```python
from build123d import *

# Parameters (mm, degrees)
POCKET001_DEPTH         = 8
FILLET_R                = 1.5
SKETCH021_R             = 2
POCKET006_DEPTH         = 8
BODY003_PLACEMENT_ANGLE = 127.1


with BuildPart() as part:
    # Sketch009 → Revolution002 (revolve)
    with BuildSketch(Plane.XZ):
        Polygon((35.8, -1.2), (0, -1.2), (0, 0), (37, 0), (37, -2.8), (37, -3.8), (42.222646, -15), (26, -15), (26, -13), (35.8, -3.2), align=None)
    revolve(axis=Axis((0, 0, 0), (0, 0, 1)))

    # Sketch010 (on Face6 of Revolution002) → Pocket001 (cut)
    with BuildSketch(Plane(origin=(0, 0, -15), x_dir=(1, 0, 0), z_dir=(0, 0, -1))):
        with BuildLine():
            ThreePointArc((-4.991228, 41.926596), (0, 37.222646), (4.991228, 41.926596))
            ThreePointArc((4.991228, 41.926596), (0, 42.222646), (-4.991228, 41.926596))
        make_face()
    extrude(amount=-POCKET001_DEPTH, mode=Mode.SUBTRACT)

    # Fillet
    fillet_edges = [part.edges().sort_by_distance(p)[0] for p in [
        (-37, 0, 0),
        (-35.8, 0, -1.2),
    ]]
    fillet(fillet_edges, radius=FILLET_R)

    # Sketch021 → Pocket006 (cut)
    with BuildSketch(Plane.XY.offset(-15)):
        with Locations((-9.025876, -28.085291)):
            Circle(SKETCH021_R)
        with Locations((26.240123, 13.479835)):
            Circle(SKETCH021_R)
        with Locations((-20.597214, 21.118825)):
            Circle(SKETCH021_R)
    extrude(amount=POCKET006_DEPTH, mode=Mode.SUBTRACT)


with BuildPart() as part_1:
    # Body003 placement: moved
    add(part.part.moved(Location((0, 0, 27.04))).rotate(Axis((0, 0, 27.04), (0, 0, 1)), BODY003_PLACEMENT_ANGLE))


solid = part_1.part
```
Source: CAD feature listing. Evaluate the final solid. Frame: model axes, mm. A direction names the side the tool comes from. Round coordinates to 2 decimals unless told otherwise and drop trailing zeros. Loops run counter-clockwise (first coordinate to the right, second up) from the corner with the lowest first, then second, coordinate; pieces in that order, holes last. Notation, with made-up numbers: (79, -6.5) - (98, -6.5) arc R21 cw to (98, 27.5) - close; hole circle Ø3 at (8.25, 32.5). An arc over 180 degrees is marked (long way). Use CSV: the item, a comma, the result in double quotes.
Q1. Pin query (flat end, axial travel): pin 1 Ø1 at (x, z) = (10, 25) entering from -Y; pin 2 Ø2 at (y, z) = (24, 24.5) entering from -X; pin 3 Ø4 at (x, y) = (14.5, -7) entering from -Z. Return the tip coordinate at first contact, or that it passes through.
Reported:
pin 1,"y = -35.76"
pin 2,"x = -28.98"
pin 3,"z = 25.84"
Q2. Ray query, line 1 along X through (y, z) = (0, 24.25); line 2 along X through (y, z) = (5, 14.25); line 3 along Y through (x, z) = (15, 22). Return the intervals inside material, ascending.
Reported:
line 1,"-37 to -35.8, 35.8 to 37"
line 2,"-40.89 to -25.73, 25.73 to 40.89"
line 3,"-34.45 to -30.47, 30.47 to 34.45"
Q3. Mould query, pull axis X, two halves, no side actions, for faces 4 (the conical face through (11.424, 24.037, 14.653)), 5 (the cylindrical face through (29.664, 10.574, 14.904)), 6 (the flat face through (30, 23, 20.04)), 7 (the cylindrical face through (-26.354, -25.97, 24.406)). Classes: pulls with the +X half, pulls with the -X half, needs draft (parallel to the pull), parting line crosses it, or undercut.
Reported:
face 4,"undercut"
face 5,"undercut"
face 6,"needs draft"
face 7,"parting line crosses it"
Q4. Section query A-A, the plane x = 0. Output: boundary loops of the cut face in (y, z), then the cut area to 3 significant figures.
Reported:
outline,"(-42.22, 12.04) - (-26, 12.04) - (-26, 14.04) - (-35.8, 23.84) - (-35.8, 24.34) arc R1.5 cw to (-34.3, 25.84) - (34.3, 25.84) arc R1.5 cw to (35.8, 24.34) - (35.8, 23.84) - (26, 14.04) - (26, 12.04) - (42.22, 12.04) - (37, 23.24) - (37, 25.54) arc R1.5 ccw to (35.5, 27.04) - (-35.5, 27.04) arc R1.5 ccw to (-37, 25.54) - (-37, 23.24) - close"
area,"316 mm^2"
Q5. Section query C-C, the plane z = 18. Output: boundary loops of the cut face in (x, y), then the cut area to 3 significant figures.
Reported:
outline,"(28.88, 26.87) arc R39.44 ccw (long way) to (33.72, 20.47) arc R5 cw to start; hole (-27.79, 11.2) arc R29.96 ccw to (-6.42, -29.26) arc R2 ccw to (-2.54, -29.85) arc R29.96 ccw to (28.87, 8.02) arc R2 ccw to (27.57, 11.72) arc R29.96 ccw to (-26.09, 14.74) arc R2 ccw to start"
area,"2,040 mm^2"
Q6. Reachability of faces 1 (the flat face through (26, -5, 12.04)), 2 (the cylindrical face through (-3.38, -35.64, 24.09)), 3 (the cylindrical face through (-4.609, -31.158, 14.904)) from +Z, -Z, +X, -X, +Y, -Y: full face, straight path, thin tool, end or side. Return the list, or none.
Reported:
face 1,"-Z, +X, -X, +Y, -Y"
face 2,"none"
face 3,"-Z"
